Autodesk Inventor part; units mm, degrees
ref_plane "Work Plane2" through (0, 0, 5) normal (0, 0, 1) x (1, 0, 0)
ref_plane "Work Plane8" through (0, 0, 0) normal (0.9238795, 0.3826834, 0) x (0, 0, 1)
ref_plane "Work Plane9" through (0, 0, 0) normal (1, 0, 0) x (0, 1, 0)
sketch "Sketch1" plane through (0, 0, 0) normal (0, 0, 1) x (1, 0, 0)
  circle A0 centre (0, 0) radius 7.8925
  dimension "d0" = 15.785
extrude "Extrusion1" add sketch "Sketch1" along normal blind 10
ref_plane "Work Plane2" through (0, 0, 5) normal (0, 0, 1) x (1, 0, 0)
sketch "Sketch2" plane through (0, 0, 0) normal (0, 0, -1) x (-1, 0, 0)
  circle A0 centre (0, 0) radius 7.8925
  circle A1 centre (0, 0) radius 6
  dimension "d3" = 12
surface extrude "Pitch Diameter" sketch "Sketch2" against normal through all shown no curves A1
ref_plane "Work Plane8" through (0, 0, 0) normal (0.9238795, 0.3826834, 0) x (0, 0, 1)
ref_plane "Work Plane9" through (0, 0, 0) normal (1, 0, 0) x (0, 1, 0)
spur gear teeth "Spur Gear" teeth 8 pitch diameter 12 tip diameter 15.785 root diameter 7 face width 10 start plane through (0, 0, 0) normal (0, 0, -1) x (-1, 0, 0)
equation "\"d0\" = da_da"
equation "\"d1\" = da_b"
equation "\"d3\" = da_d"
properties part number "Spur Gear1" material "Steel"
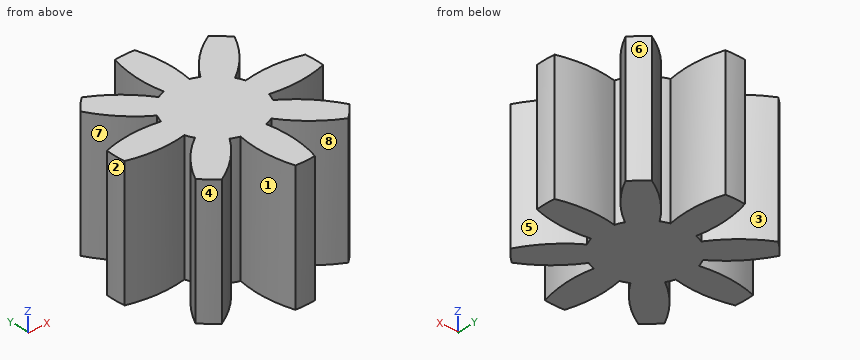
Work out the finished part from the listing and answer in its coordinate system (mm). Face numbers are marked on the shaded views. A direction names the side the tool comes from. Round coordinates to 2 decimals unless told otherwise and drop trailing zeros. Loops run counter-clockwise (first coordinate to the right, second up) from the corner with the lowest first, then second, coordinate; pieces in that order, holes last. Notation, with made-up numbers: (36, 59) - (50, 59) arc R15 ccw to (50, 78) - close; hole circle Ø2 at (35, -28). An arc over 180 degrees is marked (long way). Use one line per item in the form item = value. Start each with the question number.
(1) A flat-ended cylindrical pin translates along its axis: P1, Ø4, axis at y = 3.5, z = 1.5, coming from the -X side. Find the tip coordinate at first contact, or state that the pin passes through.
(2) Consider line 1 (Y direction, x = -4.75, z = 6.75); line 2 (Y direction, x = -6, z = 6). Determine where each line is inside the solid, lowest interval first.
(3) Find section C-C on y = -3.75. Determine the outline of the cut face in (x, z), and give its area (3 significant figures).
(4) Find section D-D on y = 2. Determine the outline of the cut face in (x, z), and give its area (3 significant figures).
(5) Find section B-B on x = 4.5. Determine the outline of the cut face in (y, z).
(6) Which of the six approach directions +Z, -Z, +X, -X, +Y, -Y give full straight-line access (tool end or side, diameter ignored) to the marked faces 1, 2, 3, 4 and 5?
(7) Determine the mould class of the marked faces 6, 7 and 8 for opening direction X: +X half, -X half, draft (parallel to the pull), parting line (faces both ways), or undercut.
Answer list:
q1.P1 = -6.1
q2.line_1 = -5.96 to -3.09, -1.18 to 1.18, 3.09 to 5.96
q2.line_2 = -5.13 to -4.82, -1.14 to 1.14, 4.82 to 5.13
q3.outline = (-5.3, 0) - (-2.14, 0) - (-2.14, 10) - (-5.3, 10) - close; (-1.08, 0) - (1.08, 0) - (1.08, 10) - (-1.08, 10) - close; (2.14, 0) - (5.3, 0) - (5.3, 10) - (2.14, 10) - close
q3.area = 84.9 mm^2
q4.outline = (-3.57, 0) - (3.57, 0) - (3.57, 10) - (-3.57, 10) - close
q4.area = 71.4 mm^2
q5.outline = (-5.81, 0) - (-2.82, 0) - (-2.82, 10) - (-5.81, 10) - close; (-1.17, 0) - (1.17, 0) - (1.17, 10) - (-1.17, 10) - close; (2.82, 0) - (5.81, 0) - (5.81, 10) - (2.82, 10) - close
q6.face_1 = +Z, -Z
q6.face_2 = +Z, -Z, -X
q6.face_3 = +Z, -Z, +Y
q6.face_4 = +Z, -Z, -X, -Y
q6.face_5 = +Z, -Z, +X
q7.face_6 = +X half
q7.face_7 = -X half
q7.face_8 = undercut
